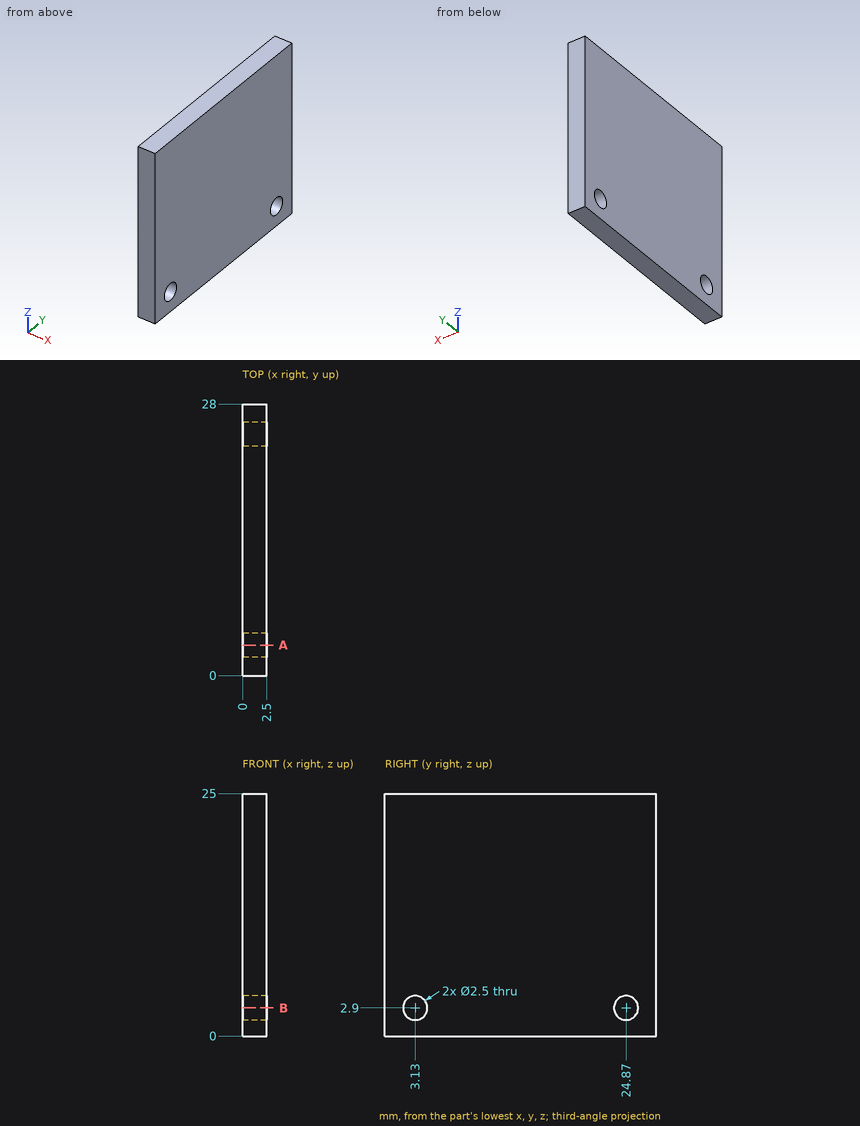
Can you work these out from the drawing? Everything is in mm from the part's minimum corner. Coordinates: 2 decimals unless noted, no trailing zeros. Loops run counter-clockwise (first coordinate to the right, second up) from the corner with the lowest first, then second, coordinate; pieces in that order, holes last. Notation, with made-up numbers: M -25.5,-31.5 L 11.5,-31.5 A12 cw 11.5,-16.5 Z; hole C 4.5,45 d8. An arc over 180 degrees is marked long. Put each result on its own line as item: value. Start each with the question number.
(1) Will this pin go through, and if not, where does the flat tip stop? P1, Ø3, axis at y = 17, z = 3.5, coming from the -X side.
(2) I need wall thicknesses on line 1 (Y direction, x = 1.6, z = 2.9); line 2 (Y direction, x = 0.85, z = 2); line 3 (Z direction, x = 2.1, y = 25.75). Which ranges of each line are inside material? Lowest first, please. Write a range as from..to.
(3) Suppose I cut it at B-B on z = 2.9. Please give me the cut outline in (x, y).
(4) Suppose I cut it at A-A on y = 3.13. Please give me the cut outline in (x, z).
Solutions:
1. P1: stops at x = 0
2. line 1: y = 0..1.88, 4.38..23.62, 26.12..28
2. line 2: y = 0..2.26, 4..24, 25.74..28
2. line 3: z = 0..2.01, 3.79..25
3. outline: M 0,0 L 2.5,0 L 2.5,1.88 L 0,1.88 Z; M 0,4.38 L 2.5,4.38 L 2.5,23.62 L 0,23.62 Z; M 0,26.12 L 2.5,26.12 L 2.5,28 L 0,28 Z
4. outline: M 0,0 L 2.5,0 L 2.5,1.65 L 0,1.65 Z; M 0,4.15 L 2.5,4.15 L 2.5,25 L 0,25 Z
